from build123d import *

# Parameters (mm, degrees)
ESQUISSE2_R             = 1.5
BOSS_EXTRU_1_DEPTH      = 6
ENL_V_MAT_EXTRU_1_DEPTH = 0.5


with BuildPart() as part:
    # Esquisse1 → Révolution1 (revolve)
    with BuildSketch(Plane(origin=(0, 0, 0), x_dir=(-1, 0, 0), z_dir=(0, 0, -1)), mode=Mode.PRIVATE) as r_volution1_sk:
        with BuildLine():
            Line((-1.8, 2.8), (-1.8, 0))
            Line((-1.8, 0), (0, 0))
            Line((0, 0), (0, 1.817822349))
            ThreePointArc((0, 1.817822349), (-0.236450397, 2.425853536), (-0.821559832, 2.714397577))
            Line((-0.821559832, 2.714397577), (-1.8, 2.8))
        make_face()
    revolve(r_volution1_sk.sketch.rotate(Axis((1.8, 0, 0), (-1, 0, 0)), 270), axis=Axis((1.8, 0, 0), (-1, 0, 0)))

    # Esquisse2 → Boss.-Extru.1 (add)
    with BuildSketch(Plane(origin=(1.8, 0, 0), x_dir=(0, 0, -1), z_dir=(1, 0, 0))):
        Circle(ESQUISSE2_R)
    extrude(amount=BOSS_EXTRU_1_DEPTH)

    # Esquisse3 → Enlèv. mat.-Extru.1 (cut, symmetric)
    with BuildSketch(Plane(origin=(0, 0, 0), x_dir=(1, 0, 0), z_dir=(0, 1, 0))):
        with BuildLine():
            Line((0, 1.817822349), (0, -1.817822349))
            ThreePointArc((0, -1.817822349), (0.236450397, -2.425853536), (0.821559832, -2.714397577))
            Line((0.821559832, -2.714397577), (1, -2.730009069))
            Line((1, -2.730009069), (1, 2.730009069))
            Line((1, 2.730009069), (0.821559832, 2.714397577))
            ThreePointArc((0.821559832, 2.714397577), (0.236450397, 2.425853536), (0, 1.817822349))
        make_face()
    extrude(amount=ENL_V_MAT_EXTRU_1_DEPTH, both=True, mode=Mode.SUBTRACT)


solid = part.part
The model under review builds one solid part; all positions refer to its coordinate system, in mm. A direction names the side the tool comes from. Round coordinates to 2 decimals unless told otherwise and drop trailing zeros. Write each loop counter-clockwise with the first axis right and the second up, starting at its lowest first coordinate (ties: lowest second). Pieces come first, ordered by that corner, then holes. Notation, with made-up numbers: M -6,77 L 28,77 A15 cw 28,87 Z; hole C 61,17.5 d11. An arc over 180 degrees is marked long. Answer as CSV lines item,"result". Start each with the question number.
Q1. Consider section B-B, the plane z = 0. Give the boundary of the cut face in (x, y).
Q2. The part is to be moulded in two halves that separate along Y. For faces 4 (the face through (4.76, 0.07, 1.5)), 5 (the face through (0.5, 0.5, 0)), 6 (the face through (0, -1, 0)), say which applies: +Y half, -Y half, draft (parallel to the pull), parting line (faces both ways), or undercut.
Q3. Wall thickness on line 1 along Z through (x, y) = (4, -0.05); line 2 along X through (y, z) = (-1.8, 0.15); line 3 along X through (y, z) = (-0.35, 2.4): over which ranges is each line inside the solid? List them lowest first.
Q4. Consider section A-A, the plane y = 0. Give the boundary of the cut face in (x, z).
Q5. Consider section D-D, the plane x = 2.5. Give the boundary of the cut face in (y, z), then the cut area to 3 significant figures.
Q6. Clearance check with flat-ended pins moving along their axes: P1, Ø0.5, axis at y = 0, z = 0.5, coming from the -X side; P2, Ø1.1, axis at x = 0.5, z = 0, coming from the -Y side; P3, Ø2, axis at x = 6.5, y = -1, coming from the -Z side. State where each tip first meets the part, or that it passes through.
Q7. Tool access review of faces 1 (the face through (1.8, -1.2, 1.2)), 2 (the face through (0, 1, 0)), 3 (the face through (0.5, -0.5, 0)): name each direction out of +Z, -Z, +X, -X, +Y, -Y from which nothing blocks a thin tool from reaching the whole face with its end or side.
Result set:
1,outline,"M 0,-1.82 A0.9 ccw 0.82,-2.71 L 1.8,-2.8 L 1.8,-1.5 L 7.8,-1.5 L 7.8,1.5 L 1.8,1.5 L 1.8,2.8 L 0.82,2.71 A0.9 ccw 0,1.82 L 0,0.5 L 1,0.5 L 1,-0.5 L 0,-0.5 Z"
2,face 4,"parting line"
2,face 5,"undercut"
2,face 6,"draft"
3,line 1,"z = -1.5 to 1.5"
3,line 2,"x = 0 to 1.8"
3,line 3,"x = 1 to 1.8"
4,outline,"M 1,-2.73 L 1.8,-2.8 L 1.8,-1.5 L 7.8,-1.5 L 7.8,1.5 L 1.8,1.5 L 1.8,2.8 L 1,2.73 Z"
5,outline,"C 0,0 d3"
5,area,"7.07 mm²"
6,P1,"stops at x = 1"
6,P2,"stops at y = -2.73"
6,P3,"stops at z = -1.5"
7,face 1,"+X"
7,face 2,"+Z, -Z, -X, +Y, -Y"
7,face 3,"+Z, -Z, -X"
